Study the drawing (mm; zero at the part's minimum x, y, z) and answer. A direction names the side the tool comes from. Coordinates: 2 decimals unless noted, no trailing zeros. Write each loop counter-clockwise with the first axis right and the second up, starting at its lowest first coordinate (ties: lowest second). Pieces come first, ordered by that corner, then holes. Notation, with made-up numbers: (-31, -12.5) - (27, -12.5) arc R29 ccw to (27, 7.5) - close; hole circle Ø7 at (-13.75, -34). An arc over 180 degrees is marked (long way). One line per item, written item: value.
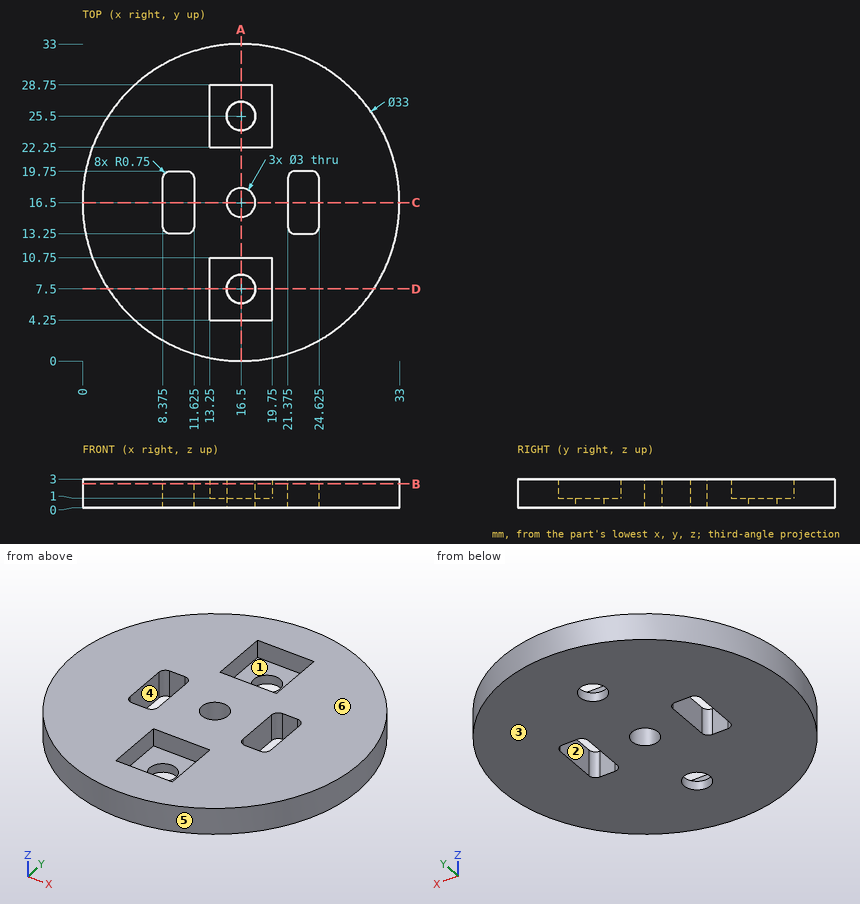
Item 1: Section B-B, the plane z = 2.5 is taken. Determine the outline of the cut face in (x, y) (3 decimals).
Evaluation:
outline: circle Ø33 at (16.5, 16.5); hole (8.375, 14) arc R0.75 ccw to (9.125, 13.25) - (10.875, 13.25) arc R0.75 ccw to (11.625, 14) - (11.625, 19) arc R0.75 ccw to (10.875, 19.75) - (9.125, 19.75) arc R0.75 ccw to (8.375, 19) - close; hole (13.25, 4.25) - (19.75, 4.25) - (19.75, 10.75) - (13.25, 10.75) - close; hole (13.25, 22.25) - (19.75, 22.25) - (19.75, 28.75) - (13.25, 28.75) - close; hole circle Ø3 at (16.5, 16.5); hole (21.375, 14) arc R0.75 ccw to (22.125, 13.25) - (23.875, 13.25) arc R0.75 ccw to (24.625, 14) - (24.625, 19) arc R0.75 ccw to (23.875, 19.75) - (22.125, 19.75) arc R0.75 ccw to (21.375, 19) - close
Item 2: Section C-C, the plane y = 16.5 is taken. Determine the outline of the cut face in (x, z) (3 decimals).
Evaluation:
outline: (0, 0) - (8.375, 0) - (8.375, 3) - (0, 3) - close; (11.625, 0) - (15, 0) - (15, 3) - (11.625, 3) - close; (18, 0) - (21.375, 0) - (21.375, 3) - (18, 3) - close; (24.625, 0) - (33, 0) - (33, 3) - (24.625, 3) - close
Item 3: Section D-D, the plane y = 7.5 is taken. Determine the outline of the cut face in (x, z), then the cut area to 3 significant figures.
Evaluation:
outline: (2.67, 0) - (15, 0) - (15, 1) - (13.25, 1) - (13.25, 3) - (2.67, 3) - close; (18, 0) - (30.33, 0) - (30.33, 3) - (19.75, 3) - (19.75, 1) - (18, 1) - close
area: 67.0 mm2
Item 4: Determine the mould class of the marked faces 4, 5 and 6 for opening direction X: +X half, -X half, draft (parallel to the pull), parting line (faces both ways), or undercut.
Evaluation:
face 4: undercut
face 5: parting line
face 6: draft
Item 5: Which of the six approach directions +Z, -Z, +X, -X, +Y, -Y give full straight-line access (tool end or side, diameter ignored) to the marked faces 1, 2 and 3?
Evaluation:
face 1: +Z
face 2: +Z, -Z
face 3: -Z, +X, -X, +Y, -Y
Item 6: Consider probe 1 along Y at (x, z) = (16.5, 0.25); probe 2 along Y at (x, z) = (16.5, 2); probe 3 along Y at (x, z) = (19.5, 1.5). Determine where each line is inside the solid, lowest interval first.
Evaluation:
probe 1: y = 0 to 6, 9 to 15, 18 to 24, 27 to 33
probe 2: y = 0 to 4.25, 10.75 to 15, 18 to 22.25, 28.75 to 33
probe 3: y = 0.28 to 4.25, 10.75 to 22.25, 28.75 to 32.72
Item 7: Section A-A, the plane x = 16.5 is taken. Determine the outline of the cut face in (y, z).
Evaluation:
outline: (0, 0) - (6, 0) - (6, 1) - (4.25, 1) - (4.25, 3) - (0, 3) - close; (9, 0) - (15, 0) - (15, 3) - (10.75, 3) - (10.75, 1) - (9, 1) - close; (18, 0) - (24, 0) - (24, 1) - (22.25, 1) - (22.25, 3) - (18, 3) - close; (27, 0) - (33, 0) - (33, 3) - (28.75, 3) - (28.75, 1) - (27, 1) - close
Item 8: Given pin 1 (1 mm diameter, centred on x = 18, z = 2, fed in from +Y); pin 2 (1.5 mm diameter, centred on y = 14.5, z = 0.5, fed in from -X); pin 3 (0.6 mm diameter, centred on y = 6.5, z = 2.5, fed in from +X); pin 4 (2.5 mm diameter, centred on x = 16.5, y = 16.5, fed in from -Z), each flat-ended and moving along its own axis, determine where each tip first touches the part or whether it passes through.
Evaluation:
pin 1: stops at y = 32.97
pin 2: stops at x = 0.05
pin 3: stops at x = 29.85
pin 4: passes through
